Verification items for the finished model (mm, model axes). Face numbers are marked on the shaded views. Coordinates: 2 decimals unless noted, no trailing zeros. Order: outer loops, then holes, each group sorted by start corner. A loop starts at its lowest first (then second) coordinate and runs counter-clockwise, first axis right, second up. Notation, with made-up numbers: M 15,72 L 38,72 A27 cw 38,104 Z; hole C 29,83 d2. An arc over 180 degrees is marked long. Return JSON: item names as keys, results as strings. Group by question number.
1. Mould release check, pull along Z, two halves, no side actions. Record for the marked faces 1, 2 and 3: +Z half, -Z half, draft (parallel to the pull), parting line (faces both ways), or undercut.
2. Gauge pin test, flat ends, axial feed: pin 1 (1 mm diameter, centred on y = 20.5, z = 7, fed in from +X); pin 2 (1.5 mm diameter, centred on x = -5, z = 5, fed in from +Y); pin 3 (10 mm diameter, centred on y = 9, z = -5.5, fed in from -X). Record the tip position at first contact, or that the pin passes through.
3. Section check A-A, the plane y = 67.5. Record the cut outline in (x, z), plus the area to 3 significant figures.
4. Material ranges on line 1 along X through (y, z) = (49, 0); line 2 along X through (y, z) = (57, 0); line 3 along Y through (x, z) = (8.5, -3), recorded low to high.
5. Section check B-B, the plane y = 24. Record the cut outline in (x, z).
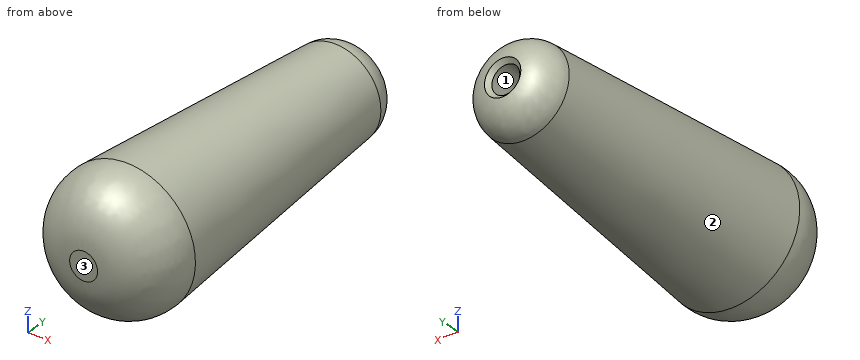
```python
from build123d import *

# Parameters (mm, degrees)
CHANFREIN1_SIZE = 1


with BuildPart() as part:
    # Esquisse1 → Révolution1 (revolve)
    with BuildSketch(Plane.XY, mode=Mode.PRIVATE) as r_volution1_sk:
        with BuildLine():
            Line((15, 12.920103162), (10, 73.644787587))
            ThreePointArc((10, 73.644787587), (7.790381776, 78.16910476), (3.1, 80))
            Line((3.1, 80), (3.1, 4))
            Line((3.1, 4), (0, 4))
            Line((0, 4), (0, 0))
            Line((0, 0), (3.1, 0))
            ThreePointArc((3.1, 0), (11.882640061, 3.851061831), (15, 12.920103162))
        make_face()
    revolve(r_volution1_sk.sketch.rotate(Axis((0, 0, 0), (0, 1, 0)), 90), axis=Axis((0, 0, 0), (0, 1, 0)))

    # Chanfrein1
    # the kernel refuses this chamfer: 1 mm, written as the material it takes off along each edge
    with BuildSketch(Plane(origin=(0, 80, 0), x_dir=(0, 0, -1), z_dir=(1, 0, 0))) as chanfrein1_piece_1:
        with BuildLine():
            Line((4.036384624, -0.063615376), (3.1, -CHANFREIN1_SIZE))
            Line((3.1, -CHANFREIN1_SIZE), (3.1, 0))
            ThreePointArc((3.1, 0), (3.582393079, -0.016826116), (4.036384624, -0.063615376))
        make_face()
    revolve(axis=Axis((0, 80, 0), (0, 1, 0)), mode=Mode.SUBTRACT)


solid = part.part
```
Answers follow:
{
 "1": {"face 1": "undercut", "face 2": "parting line", "face 3": "draft"},
 "2": {"pin 1": "x = 12.83", "pin 2": "y = 79.21", "pin 3": "x = -14.99"},
 "3": {"outline": "C 0,0 d21.01; hole C 0,0 d6.2", "area": "317 mm^2"},
 "4": {"line 1": "-12.03 to -3.1, 3.1 to 12.03", "line 2": "-11.37 to -3.1, 3.1 to 11.37", "line 3": "1.57 to 76.68"},
 "5": {"outline": "C 0,0 d28.18; hole C 0,0 d6.2"}
}
